The listing builds one solid part. Answer for the finished solid, in the listing's coordinates (mm). A direction names the side the tool comes from. Give positions to 0.01 mm unless a question says otherwise; leave off trailing zeros. Order: outer loops, then holes, each group sorted by start corner. A loop starts at its lowest first (then second) coordinate and runs counter-clockwise, first axis right, second up.
```python
from build123d import *

# Parameters (mm, degrees)
SKETCH_1_W          = 174
SKETCH_1_H          = 80
EXTRUDE_1_DEPTH     = 4
SKETCH_3_W          = 4
SKETCH_3_H          = 20
CUT_EXTRUDE_1_DEPTH = 4
SKETCH_4_W          = 50
SKETCH_4_H          = 4
CUT_EXTRUDE_2_DEPTH = 4
SKETCH_5_W          = 2
SKETCH_5_H          = 80
CUT_EXTRUDE_3_DEPTH = 10
SKETCH_8_W          = 50
SKETCH_8_H          = 4
CUT_EXTRUDE_4_DEPTH = 4
SKETCH_9_W          = 55
SKETCH_9_H          = 23.130254534
CUT_EXTRUDE_5_DEPTH = 4


with BuildPart() as part:
    # 스케치1 → 보스-돌출1 (new body)
    with BuildSketch(Plane(origin=(0, 0, 0), x_dir=(0, 0, -1), z_dir=(1, 0, 0))):
        Rectangle(SKETCH_1_W, SKETCH_1_H)
    extrude(amount=EXTRUDE_1_DEPTH)

    # 스케치3 → 컷-돌출1 (cut)
    with BuildSketch(Plane(origin=(4, 0, 0), x_dir=(0, 0, -1), z_dir=(1, 0, 0))):
        with Locations((85, 30)):
            Rectangle(SKETCH_3_W, SKETCH_3_H)
        with Locations((85, -30)):
            Rectangle(SKETCH_3_W, SKETCH_3_H)
    extrude(amount=-CUT_EXTRUDE_1_DEPTH, mode=Mode.SUBTRACT)

    # 스케치4 → 컷-돌출2 (cut)
    with BuildSketch(Plane(origin=(4, 0, 0), x_dir=(0, 0, -1), z_dir=(1, 0, 0))):
        with Locations((-2, 38)):
            Rectangle(SKETCH_4_W, SKETCH_4_H)
    extrude(amount=-CUT_EXTRUDE_2_DEPTH, mode=Mode.SUBTRACT)

    # 스케치5 → 컷-돌출3 (cut)
    with BuildSketch(Plane.ZY):
        with Locations((86, 0)):
            Rectangle(SKETCH_5_W, SKETCH_5_H)
    extrude(amount=-CUT_EXTRUDE_3_DEPTH, mode=Mode.SUBTRACT)

    # 스케치8 → 컷-돌출4 (cut)
    with BuildSketch(Plane.ZY):
        with Locations((3, -6)):
            Rectangle(SKETCH_8_W, SKETCH_8_H)
    extrude(amount=-CUT_EXTRUDE_4_DEPTH, mode=Mode.SUBTRACT)

    # 스케치9 → 컷-돌출5 (cut)
    with BuildSketch(Plane.ZY):
        with Locations((-19.5, 14.565127267)):
            Rectangle(SKETCH_9_W, SKETCH_9_H)
    extrude(amount=-CUT_EXTRUDE_5_DEPTH, mode=Mode.SUBTRACT)


solid = part.part
```
1) A tool of negligible diameter and unlimited length cuts with its end or side. For faces 5 (the flat face through (2, -6, -22)), 6 (the flat face through (2, 36, 2)), 7 (the flat face through (2, 20, -85)), from which of +Z, -Z, +X, -X, +Y, -Y can it reach the whole face along a straight path? Write none if from no direction.
Geometry says:
face 5: +X, -X
face 6: +X, -X, +Y
face 7: -Z, +X, -X, +Y
2) Find section A-A (z = 14). Write down the section's boundary in (x, y), then the cut area to 3 significant figures.
Geometry says:
outline: (0, -40) - (4, -40) - (4, -8) - (0, -8) - close; (0, -4) - (4, -4) - (4, 36) - (0, 36) - close
area: 288 mm2
3) For a pull along Z with two mould halves and no side action, classify faces 1 (the flat face through (2, 3, -20)), 2 (the flat face through (2, 40, -53)), 3 (the flat face through (2, 30, -83)), 4 (the flat face through (2, 14, -47)) as +Z half, -Z half, draft (parallel to the pull), parting line (faces both ways), or undercut.
Geometry says:
face 1: undercut
face 2: draft
face 3: -Z half
face 4: undercut
4) Straight lines are drawn through the part: probe 1 along Y at (x, z) = (2.4, -20); probe 2 along Y at (x, z) = (2.45, -44.5); probe 3 along Y at (x, z) = (1.1, 24.5). For each, find the intervals that lie inside material, in ascending order.
Geometry says:
probe 1: y = -40 to -8, -4 to 3, 26.13 to 36
probe 2: y = -40 to 3, 26.13 to 40
probe 3: y = -40 to -8, -4 to 36
5) Given P1, Ø1.2, axis at x = 2.5, y = 28.5, coming from the -Z side; P2, Ø2, axis at x = 1, z = -5, coming from the +Y side; P3, Ø1.2, axis at x = 3, z = -85.5, coming from the +Y side, each flat-ended and moving along its own axis, determine where each tip first touches the part or whether it passes through.
Geometry says:
P1: stops at z = -83
P2: stops at y = 36
P3: stops at y = 20
6) Find section D-D (z = -44). Write down the section's boundary in (x, y).
Geometry says:
outline: (0, -40) - (4, -40) - (4, 3) - (0, 3) - close; (0, 26.13) - (4, 26.13) - (4, 40) - (0, 40) - close
7) Find section C-C (y = -31.5). Write down the section's boundary in (x, z), then the cut area to 3 significant figures.
Geometry says:
outline: (0, -83) - (4, -83) - (4, 85) - (0, 85) - close
area: 672 mm2
8) Find section B-B (x = 1.95). Write down the section's boundary in (y, z), then the cut area to 3 significant figures.
Geometry says:
outline: (-40, -83) - (-20, -83) - (-20, -87) - (20, -87) - (20, -83) - (40, -83) - (40, -23) - (36, -23) - (36, 27) - (40, 27) - (40, 85) - (-40, 85) - close; hole (-8, -22) - (-4, -22) - (-4, 28) - (-8, 28) - close; hole (3, -47) - (26.13, -47) - (26.13, 8) - (3, 8) - close
area: 11,900 mm2
